Could you check a few things on this drawing? It's one solid part, dimensions in mm from its lowest x, y, z. Give positions to 0.01 mm unless a question says otherwise; leave off trailing zeros. Order: outer loops, then holes, each group sorted by start corner. A loop starts at its lowest first (then second) coordinate and runs counter-clockwise, first axis right, second up. Notation, with made-up numbers: M 52,70 L 105,70 A27 ccw 105,94 Z; hole C 2.5,64 d7. An arc over 180 degrees is marked long. One line per item, written item: value. Start each with the question number.
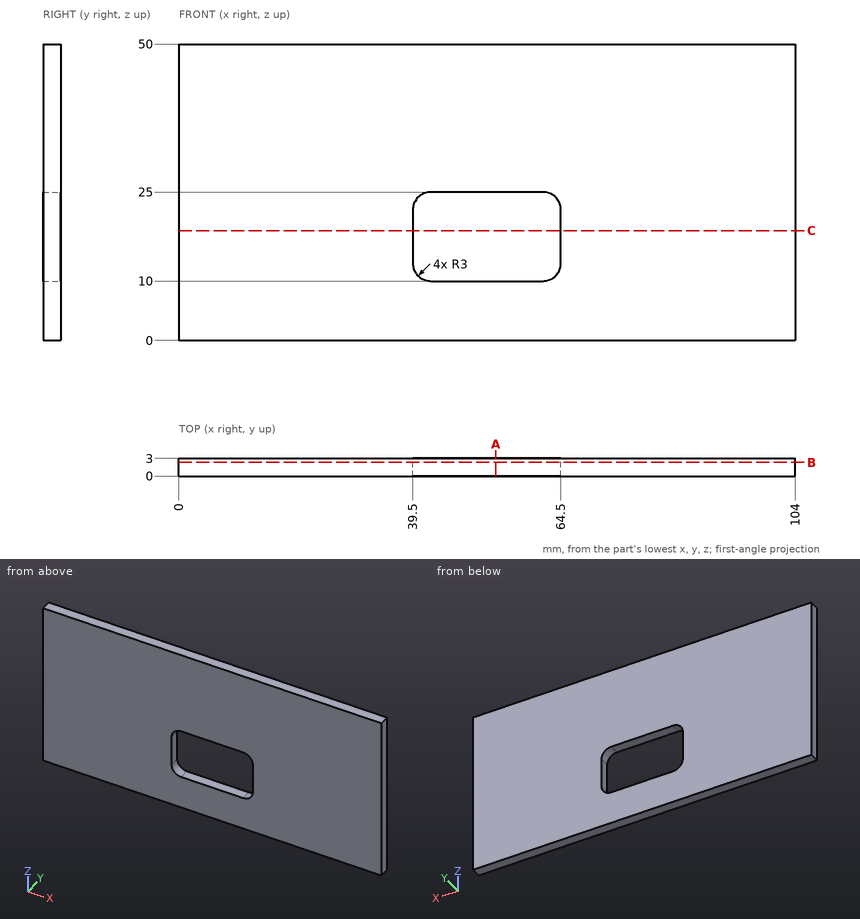
Item 1: Please list where these lines run through material, in increasing order: probe 1 along Z at (x, y) = (45.5, 0.8); probe 2 along X at (y, z) = (0.4, 16); probe 3 along X at (y, z) = (2.95, 23). Write a range as [from, to].
Item 2: I want a section at B-B on y = 2.3. Write out the boundary of the cut face in (x, z).
Item 3: I want a section at A-A on x = 53.5. Write out the boundary of the cut face in (y, z).
Item 4: I want a section at C-C on z = 18.5. Write out the boundary of the cut face in (x, y), plus the area to 3 significant figures.
Answer below:
1. probe 1: z = [0, 10], [25, 50]
1. probe 2: x = [0, 39.5], [64.5, 104]
1. probe 3: x = [0, 39.67], [64.33, 104]
2. outline: M 0,0 L 104,0 L 104,50 L 0,50 Z; hole M 39.5,13 A3 ccw 42.5,10 L 61.5,10 A3 ccw 64.5,13 L 64.5,22 A3 ccw 61.5,25 L 42.5,25 A3 ccw 39.5,22 Z
3. outline: M 0,0 L 3,0 L 3,10 L 0,10 Z; M 0,25 L 3,25 L 3,50 L 0,50 Z
4. outline: M 0,0 L 39.5,0 L 39.5,3 L 0,3 Z; M 64.5,0 L 104,0 L 104,3 L 64.5,3 Z
4. area: 237 mm²
